from build123d import *

# Parameters (mm, degrees)
EXTRUDE_1_DEPTH                 = 1.5
BOSS_EXTRUDE3_REACH             = 24.677
BOSS_EXTRUDE3_DIRECTION_2_REACH = 24.677


with BuildPart() as part:
    # Эскиз1 → Бобышка-Вытянуть1 (new, symmetric)
    with BuildSketch(Plane.XY):
        with BuildLine():
            ThreePointArc((5, -15.198684154), (15.454813221, -4.141104722), (11.929469096, 10.662446581))
            ThreePointArc((11.929469096, 10.662446581), (-15.454813221, 4.141104722), (5, -15.198684154))
        make_face()
        with BuildLine():
            Line((-2.5, -2.359609465), (-2.5, -3.304777846))
            ThreePointArc((-2.5, -3.304777846), (0, -12.85), (2.5, -3.304777846))
            Line((2.5, -3.304777846), (2.5, -2.359609465))
            ThreePointArc((2.5, -2.359609465), (4.180016715, -1.604605606), (5.649137352, -0.493672869))
            Line((5.649137352, -0.493672869), (6.41139529, -0.943209602))
            ThreePointArc((6.41139529, -0.943209602), (12.678644072, -2.027149068), (8.69732788, 2.932936963))
            Line((8.69732788, 2.932936963), (7.935069942, 3.382473696))
            ThreePointArc((7.935069942, 3.382473696), (0, 13.65), (-7.935069942, 3.382473696))
            Line((-7.935069942, 3.382473696), (-8.69732788, 2.932936963))
            ThreePointArc((-8.69732788, 2.932936963), (-12.678644072, -2.027149068), (-6.41139529, -0.943209602))
            Line((-6.41139529, -0.943209602), (-5.649137352, -0.493672869))
            ThreePointArc((-5.649137352, -0.493672869), (-4.180016715, -1.604605606), (-2.5, -2.359609465))
        make_face(mode=Mode.SUBTRACT)
    extrude(amount=EXTRUDE_1_DEPTH, both=True)

    # Boss-Extrude3: up to this face of the body (flat: up to its plane)
    boss_extrude3_end = Plane(part.part.faces().sort_by_distance((15.017685091, -4.023976592, 1.5))[0])
    # Sketch2 → Boss-Extrude3 (add, up to the picked face)
    with BuildSketch(Plane.XY, mode=Mode.PRIVATE) as boss_extrude3_sk1:
        with BuildLine():
            ThreePointArc((13.856406461, 8), (0, -16), (-13.856406461, 8))
            Line((-13.856406461, 8), (-14.722431864, 8.5))
            ThreePointArc((-14.722431864, 8.5), (-15.822781238, -6.216075442), (-5, -16.248076809))
            ThreePointArc((-5, -16.248076809), (13.294669863, -10.59489279), (14.722431864, 8.5))
            Line((14.722431864, 8.5), (13.856406461, 8))
        make_face()
    boss_extrude3_tool1 = split(extrude(boss_extrude3_sk1.sketch, amount=BOSS_EXTRUDE3_REACH, mode=Mode.PRIVATE), bisect_by=boss_extrude3_end, keep=Keep.BOTH, mode=Mode.PRIVATE)
    add(boss_extrude3_tool1.solids().sort_by(Axis((14.501919, 7.881939, 0), (0, 0, 1)))[0])

    # Boss-Extrude3 direction 2: up to this face of the body (flat: up to its plane)
    boss_extrude3_direction_2_end = Plane(part.part.faces().sort_by_distance((15.017685091, -4.023976592, -1.5))[0])
    # Sketch2 → Boss-Extrude3 direction 2 (add, up to the picked face)
    with BuildSketch(Plane.XY, mode=Mode.PRIVATE) as boss_extrude3_direction_2_sk1:
        with BuildLine():
            ThreePointArc((13.856406461, 8), (0, -16), (-13.856406461, 8))
            Line((-13.856406461, 8), (-14.722431864, 8.5))
            ThreePointArc((-14.722431864, 8.5), (-15.822781238, -6.216075442), (-5, -16.248076809))
            ThreePointArc((-5, -16.248076809), (13.294669863, -10.59489279), (14.722431864, 8.5))
            Line((14.722431864, 8.5), (13.856406461, 8))
        make_face()
    boss_extrude3_direction_2_tool1 = split(extrude(boss_extrude3_direction_2_sk1.sketch, amount=-BOSS_EXTRUDE3_DIRECTION_2_REACH, mode=Mode.PRIVATE), bisect_by=boss_extrude3_direction_2_end, keep=Keep.BOTH, mode=Mode.PRIVATE)
    add(boss_extrude3_direction_2_tool1.solids().sort_by(Axis((14.501919, 7.881939, 0), (0, 0, -1)))[0])


solid = part.part
Geometry: final body of the model. Coordinates: model frame, mm. A direction names the side the tool comes from. Give positions to 0.01 mm unless a question says otherwise; leave off trailing zeros. Order: outer loops, then holes, each group sorted by start corner. A loop starts at its lowest first (then second) coordinate and runs counter-clockwise, first axis right, second up. Notation, with made-up numbers: (78, 20.25) - (107, 20.25) arc R24 cw to (107, 35.25) - close; hole circle Ø6 at (-6, -1). An arc over 180 degrees is marked (long way). Use CSV: the item, a comma, the result in double quotes.
1. Access query for faces 4 (the face through (-2.5, -3, 0)), 5 (the face through (-14.283, 8.246, 0.021)), 6 (the face through (-4, -4, -1.5)). Directions: +Z, -Z, +X, -X, +Y, -Y. A direction counts if a zero-diameter tool reaches every point of the face in a straight line with its end or side. Return the directions, or none.
Answers below:
face 4,"+Z, -Z"
face 5,"+Z, -Z, +Y"
face 6,"-Z, +X, -X, +Y, -Y"
2. Section query B-B (z = 0.9). Output: boundary loops of the cut face in (x, y).
Answers below:
outline,"(-14.72, 8.5) arc R17 ccw (long way) to (14.72, 8.5) - (13.86, 8) arc R16 ccw to (-13.86, 8) - close; hole (-8.7, 2.93) arc R3.4 ccw (long way) to (-6.41, -0.94) - (-5.65, -0.49) arc R8.2 ccw to (-2.5, -2.36) - (-2.5, -3.3) arc R5.1 ccw (long way) to (2.5, -3.3) - (2.5, -2.36) arc R8.2 ccw to (5.65, -0.49) - (6.41, -0.94) arc R3.4 ccw (long way) to (8.7, 2.93) - (7.94, 3.38) arc R8.2 ccw (long way) to (-7.94, 3.38) - close"
3. Section query C-C (y = 0). Output: boundary loops of the cut face in (x, z), plus the area to 3 significant figures.
Answers below:
outline,"(-17, -1.5) - (-13.14, -1.5) - (-13.14, 1.5) - (-17, 1.5) - close; (13.14, -1.5) - (17, -1.5) - (17, 1.5) - (13.14, 1.5) - close"
area,"23.2 mm2"
4. Mould query, pull axis Y, two halves, no side actions, for faces 1 (the face through (14.295, 8.254, 0.021)), 2 (the face through (0, -17, 0)), 3 (the face through (2.5, -3, 0)). Classes: +Y half, -Y half, draft (parallel to the pull), parting line (faces both ways), or undercut.
Answers below:
face 1,"+Y half"
face 2,"parting line"
face 3,"undercut"
5. Section query A-A (x = 0). Output: boundary loops of the cut face in (y, z).
Answers below:
outline,"(-17, -1.5) - (-12.85, -1.5) - (-12.85, 1.5) - (-17, 1.5) - close; (13.65, -1.5) - (16, -1.5) - (16, 1.5) - (13.65, 1.5) - close"
6. Contact query for flat-ended pins moving along their axis: pin 1 (1 mm diameter, centred on x = 1, z = 0, fed in from -Y); pin 2 (0.5 mm diameter, centred on y = -2.5, z = 0.5, fed in from +X); pin 3 (13 mm diameter, centred on x = 0, y = 5.45, fed in from -Z); pin 4 (1 mm diameter, centred on y = -3, z = 0, fed in from -X). Output: stop coordinate, or through.
Answers below:
pin 1,"y = -16.99"
pin 2,"x = 16.85"
pin 3,"through"
pin 4,"x = -16.82"
7. Material intervals for line 1 along X through (y, z) = (-1, -0.15); line 2 along Y through (x, z) = (-9.75, 0); line 3 along X through (y, z) = (-7.75, -0.65), sorted ascending. Write a range as from..to.
Answers below:
line 1,"-16.97..-13.08, -6.42..-5.06, 5.06..6.42, 13.08..16.97"
line 2,"-13.93..-3.7, 3.1..12.69"
line 3,"-15.13..-5.1, 5.1..15.13"
8. Section query D-D (x = -4). Output: boundary loops of the cut face in (y, z), plus the area to 3 significant figures.
Answers below:
outline,"(-16.52, -1.5) - (-10.91, -1.5) - (-10.91, 1.5) - (-16.52, 1.5) - close; (-4.59, -1.5) - (-1.71, -1.5) - (-1.71, 1.5) - (-4.59, 1.5) - close; (12.61, -1.5) - (15.49, -1.5) - (15.49, 1.5) - (12.61, 1.5) - close"
area,"34.1 mm2"
